Geometry check sheet. Reference: drawing and pictorial views, mm from the part's lowest x, y, z. Round coordinates to 2 decimals unless told otherwise and drop trailing zeros. Order: outer loops, then holes, each group sorted by start corner. A loop starts at its lowest first (then second) coordinate and runs counter-clockwise, first axis right, second up.
(1) Sectioned sample at D-D (x = 76). Record the boundary of the cut face in (y, z), plus the area to 3 significant figures.
(2) Sectioned sample at B-B (z = 3.05). Record the boundary of the cut face in (x, y), plus the area to 3 significant figures.
(3) Sectioned sample at A-A (x = 32.66). Record the boundary of the cut face in (y, z).
(4) Material ranges on line 1 along Y through (x, z) = (32.66, 1.55); line 2 along Y through (x, z) = (50, 4.9); line 3 along Z through (x, y) = (15, 4.25), recorded low to high.
(5) Go/stop test with a flat-tipped pin: pin 1 (1.5 mm diameter, centred on y = 7, z = 1.5, fed in from +X). Record where the tip stops, or that it passes through.
(6) Release check for a two-part mould opening along Y. For the marked faces 1, 2 and 3 record: +Y half, -Y half, draft (parallel to the pull), parting line (faces both ways), or undercut.
(7) Sectioned sample at C-C (y = 20). Record the boundary of the cut face in (x, z), plus the area to 3 significant figures.
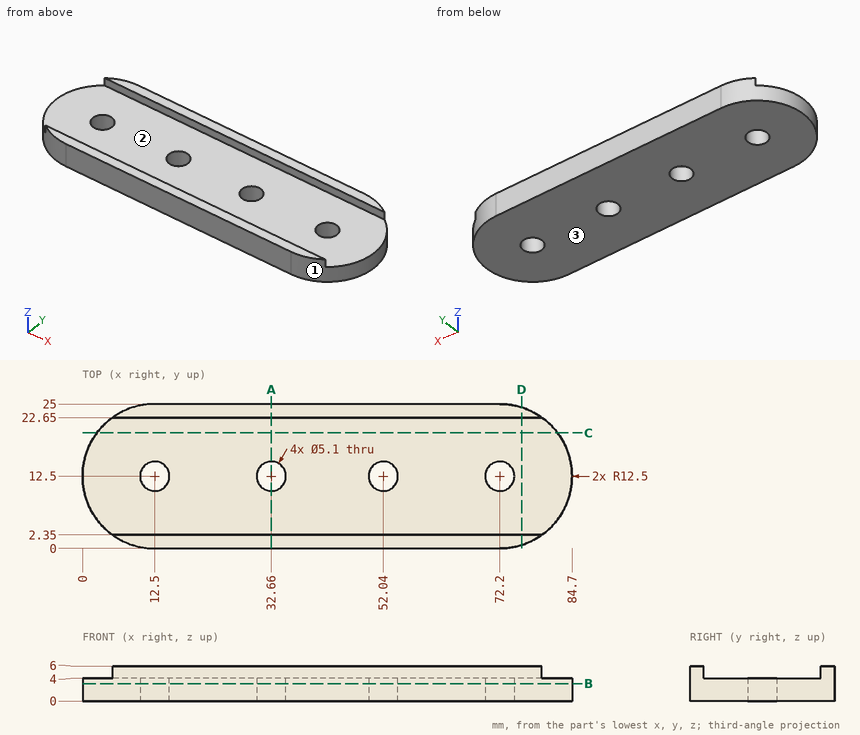
Answer below:
1. outline: (0.59, 0) - (24.41, 0) - (24.41, 6) - (22.65, 6) - (22.65, 4) - (2.35, 4) - (2.35, 6) - (0.59, 6) - close
1. area: 102 mm2
2. outline: (12.5, 0) - (72.2, 0) arc R12.5 ccw to (72.2, 25) - (12.5, 25) arc R12.5 ccw to start; hole circle Ø5.1 at (12.5, 12.5); hole circle Ø5.1 at (32.66, 12.5); hole circle Ø5.1 at (52.04, 12.5); hole circle Ø5.1 at (72.2, 12.5)
2. area: 1,900 mm2
3. outline: (0, 0) - (9.95, 0) - (9.95, 4) - (2.35, 4) - (2.35, 6) - (0, 6) - close; (15.05, 0) - (25, 0) - (25, 6) - (22.65, 6) - (22.65, 4) - (15.05, 4) - close
4. line 1: y = 0 to 9.95, 15.05 to 25
4. line 2: y = 0 to 2.35, 22.65 to 25
4. line 3: z = 0 to 4
5. pin 1: stops at x = 83.76
6. face 1: parting line
6. face 2: undercut
6. face 3: draft
7. outline: (2.5, 0) - (82.2, 0) - (82.2, 4) - (2.5, 4) - close
7. area: 319 mm2
